```python
from build123d import *

# Parameters (mm, degrees)
SKETCH1_R             = 7.5
BOSS_EXTRUDE1_DEPTH   = 5
SKETCH3_R             = 20
BOSS_EXTRUDE2_DEPTH   = 20
SKETCH4_R             = 15
BOSS_EXTRUDE3_DEPTH   = 10
SKETCH5_R             = 20
BOSS_EXTRUDE4_DEPTH   = 5
BODY_MOVE_COPY1_ANGLE = 90


with BuildPart() as part:
    # Sketch1 → Boss-Extrude1 (new body)
    with BuildSketch(Plane(origin=(0, 0, 0), x_dir=(1, 0, 0), z_dir=(0, 1, 0))):
        with BuildLine():
            ThreePointArc((-39.749220484, 58.127463165), (-58.377062168, 58.381791069), (-58.131919931, 39.753826237))
            ThreePointArc((-58.131919931, 39.753826237), (-40.976062677, -0.15633362), (-58.131919931, -40.066493476))
            ThreePointArc((-58.131919931, -40.066493476), (-58.377062168, -58.694458308), (-39.749220484, -58.440130404))
            ThreePointArc((-39.749220484, -58.440130404), (0.58615995, -41.266091018), (40.663235765, -59.034561344))
            ThreePointArc((40.663235765, -59.034561344), (58.984188278, -58.390820393), (58.444979195, -40.066493476))
            ThreePointArc((58.444979195, -40.066493476), (41.289121941, -0.15633362), (58.444979195, 39.753826237))
            ThreePointArc((58.444979195, 39.753826237), (58.984188278, 58.078153154), (40.663235765, 58.721894105))
            ThreePointArc((40.663235765, 58.721894105), (0.58615995, 40.953423779), (-39.749220484, 58.127463165))
        make_face()
        with Locations(Location((-49.186940736, 49.187136748, 0), (0, 0, 270))):
            Circle(SKETCH1_R, mode=Mode.SUBTRACT)
        with Locations(Location((49.5, 49.187136748, 0), (0, 0, 270))):
            Circle(SKETCH1_R, mode=Mode.SUBTRACT)
        with Locations(Location((-49.186940736, -49.499803987, 0), (0, 0, 270))):
            Circle(SKETCH1_R, mode=Mode.SUBTRACT)
        with Locations(Location((49.5, -49.499803987, 0), (0, 0, 270))):
            Circle(SKETCH1_R, mode=Mode.SUBTRACT)
    extrude(amount=BOSS_EXTRUDE1_DEPTH)

    # Sketch3 → Boss-Extrude2 (add)
    with BuildSketch(Plane(origin=(0, 5, 0), x_dir=(1, 0, 0), z_dir=(0, 1, 0))):
        with Locations(Location((0, 0, 0), (0, 0, 270))):
            Circle(SKETCH3_R)
    extrude(amount=BOSS_EXTRUDE2_DEPTH)

    # Sketch4 → Boss-Extrude3 (add)
    with BuildSketch(Plane(origin=(0, 25, 0), x_dir=(1, 0, 0), z_dir=(0, 1, 0))):
        with Locations(Location((0, 0, 0), (0, 0, 270))):
            Circle(SKETCH4_R)
    extrude(amount=BOSS_EXTRUDE3_DEPTH)

    # Sketch5 → Boss-Extrude4 (add)
    with BuildSketch(Plane(origin=(0, 35, 0), x_dir=(1, 0, 0), z_dir=(0, 1, 0))):
        with Locations(Location((0, 0, 0), (0, 0, 270))):
            Circle(SKETCH5_R)
    extrude(amount=BOSS_EXTRUDE4_DEPTH)


with BuildPart() as part_1:
    # Body-Move/Copy1: read off the stored shape, not the designer's step
    # Body-Move/Copy1: moved
    add(part.part.moved(Location((0, -25, 0))).rotate(Axis((0, 0, 0), (1, 0, 0)), BODY_MOVE_COPY1_ANGLE))


solid = part_1.part
```
Design review of the part built by this model. Coordinates are the model's own, in mm. A direction names the side the tool comes from. Coordinates: 2 decimals unless noted, no trailing zeros. Order: outer loops, then holes, each group sorted by start corner. A loop starts at its lowest first (then second) coordinate and runs counter-clockwise, first axis right, second up.
1) Mouldability with a two-part tool opening along Z and no side actions: class faces 4 (the flat face through (0, 0, 15)), 5 (the flat face through (-1, 1, -25)), 6 (the flat face through (15, -3, 10)), 7 (the cylindrical face through (58.787, -58.596, -22.535)) as +Z half, -Z half, draft (parallel to the pull), parting line (faces both ways), or undercut.
2) Clearance check with flat-ended pins moving along their axes: pin 1 (6 mm diameter, centred on x = -13.5, z = 1, fed in from +Y) (3 decimals); pin 2 (4 mm diameter, centred on x = 19.5, z = -6, fed in from -Y); pin 3 (2 mm diameter, centred on x = -25.5, y = 35, fed in from +Z); pin 4 (9 mm diameter, centred on x = 49.5, y = 49.19, fed in from -Z). State where each tip first meets the part, or that it passes through.
3) Wall thickness on line 1 along Y through (x, z) = (49, -23); line 2 along Z through (x, y) = (18.5, 23.5); line 3 along Z through (x, y) = (-17.5, 0): over which ranges is each line inside the solid? List them lowest first.
4) Take a section at A-A, the plane y = -46. Give the boundary of the cut face in (x, z).
5) Take a section at D-D, the plane x = 0. Give the boundary of the cut face in (y, z), and give its area (3 significant figures).
6) Take a section at B-B, the plane x = 49.5. Give the boundary of the cut face in (y, z), and give its area (3 significant figures).
7) For faces 1 (the cylindrical face through (0.88, 19.98, -10.14)), 2 (the cylindrical face through (1.22, 40.96, -22.54)), 3 (the cylindrical face through (0.66, 14.985, 4.93)), list the 3-axis set-ups (+Z, -Z, +X, -X, +Y, -Y) from which the entire face can be reached by the end or side of a thin tool; tool diameter is ignored.
8) Take a section at C-C, the plane z = -22. Give the boundary of the cut face in (x, y), and give its area (3 significant figures).
Returned:
1. face 4: +Z half
1. face 5: -Z half
1. face 6: undercut
1. face 7: draft
2. pin 1: stops at y = 16.915
2. pin 2: stops at y = -9.68
2. pin 3: stops at z = -20
2. pin 4: passes through
3. line 1: y = -62.49 to -56.98, -42.02 to -28.24, 27.93 to 41.7, 56.67 to 62.18
3. line 2: z = -25 to -20
3. line 3: z = -25 to 0, 10 to 15
4. outline: (-61.71, -25) - (-55.82, -25) - (-55.82, -20) - (-61.71, -20) - close; (-42.55, -25) - (-22.15, -25) - (-22.15, -20) - (-42.55, -20) - close; (22.51, -25) - (42.87, -25) - (42.87, -20) - (22.51, -20) - close; (56.13, -25) - (62.02, -25) - (62.02, -20) - (56.13, -20) - close
5. outline: (-41.26, -25) - (40.95, -25) - (40.95, -20) - (20, -20) - (20, 0) - (15, 0) - (15, 10) - (20, 10) - (20, 15) - (-20, 15) - (-20, 10) - (-15, 10) - (-15, 0) - (-20, 0) - (-20, -20) - (-41.26, -20) - close
5. area: 1,710 mm2
6. outline: (-62.5, -25) - (-57, -25) - (-57, -20) - (-62.5, -20) - close; (-42, -25) - (-29.07, -25) - (-29.07, -20) - (-42, -20) - close; (28.75, -25) - (41.69, -25) - (41.69, -20) - (28.75, -20) - close; (56.69, -25) - (62.19, -25) - (62.19, -20) - (56.69, -20) - close
6. area: 184 mm2
7. face 1: +Z
7. face 2: +Z, -Z, +Y
7. face 3: none
8. outline: (-58.13, -40.07) arc R13 ccw (long way) to (-39.75, -58.44) arc R55 cw to (40.66, -59.03) arc R13 ccw to (58.44, -40.07) arc R55 cw to (58.44, 39.75) arc R13 ccw to (40.66, 58.72) arc R55 cw to (-39.75, 58.13) arc R13 ccw (long way) to (-58.13, 39.75) arc R55 cw to start; hole circle Ø15 at (-49.19, -49.5); hole circle Ø15 at (-49.19, 49.19); hole circle Ø15 at (49.5, -49.5); hole circle Ø15 at (49.5, 49.19)
8. area: 9,520 mm2
